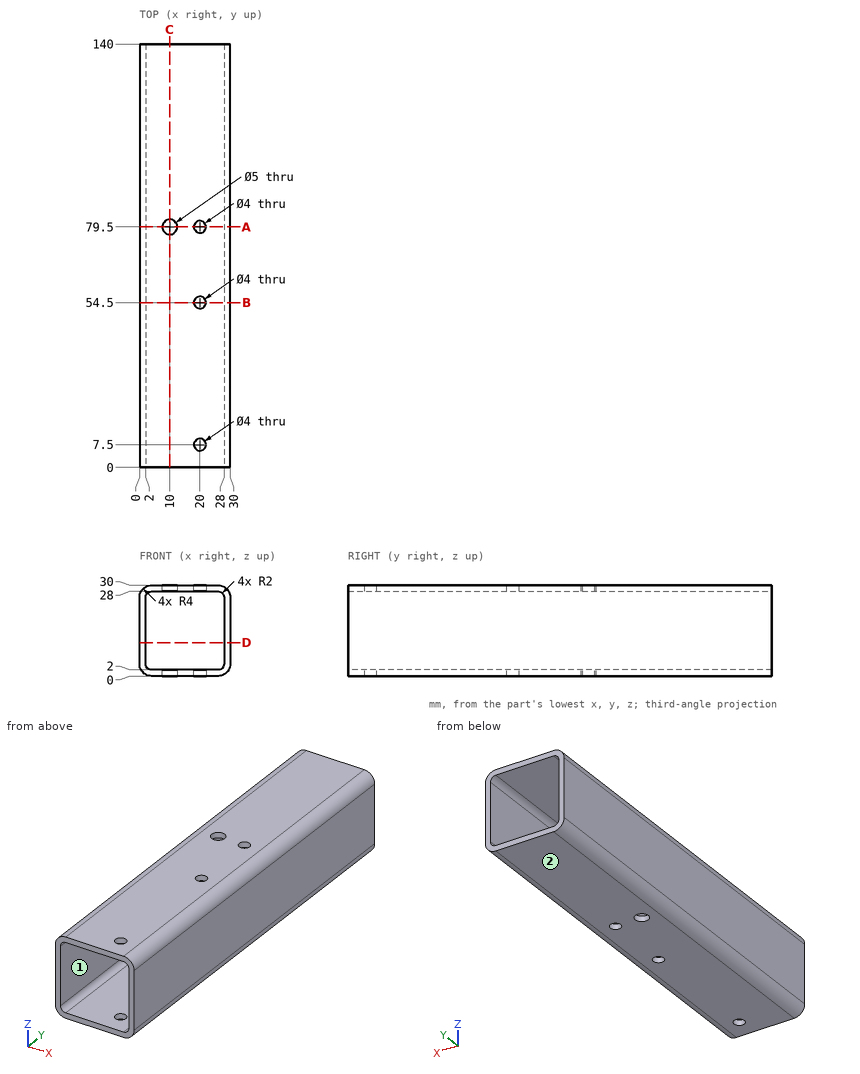
Job drawing, mm, ordinate dimensions from the low corner. One solid piece. A direction names the side the tool comes from. Give positions to 0.01 mm unless a question says otherwise; leave off trailing zeros. Write each loop counter-clockwise with the first axis right and the second up, starting at its lowest first coordinate (ties: lowest second). Pieces come first, ordered by that corner, then holes. Notation, with made-up numbers: (33, 3.25) -> (43, 3.25) arc R9 ccw to (43, 10.25) -> close; hole circle Ø1 at (9.25, -5). An arc over 180 degrees is marked (long way). Return JSON: item names as keys, results as strings.
Item 1: Band-saw the part on D-D (z = 11). List the corners of the cut face in (x, y).
Answer below:
{"outline": "(0, 0) -> (2, 0) -> (2, 140) -> (0, 140) -> close; (28, 0) -> (30, 0) -> (30, 140) -> (28, 140) -> close"}
Item 2: Drill centre lines: probe 1 along Y at (x, z) = (20, 29.25); probe 2 along Y at (x, z) = (10, 29.1); probe 3 along Z at (x, y) = (10.5, 38). Where is each one in solid material? Low to high.
Answer below:
{"probe 1": "y = 0 to 5.5, 9.5 to 52.5, 56.5 to 77.5, 81.5 to 140", "probe 2": "y = 0 to 77, 82 to 140", "probe 3": "z = 0 to 2, 28 to 30"}
Item 3: Band-saw the part on B-B (y = 54.5). List the corners of the cut face in (x, z), then the cut area to 3 significant figures.
Answer below:
{"outline": "(0, 4) arc R4 ccw to (4, 0) -> (18, 0) -> (18, 2) -> (4, 2) arc R2 cw to (2, 4) -> (2, 26) arc R2 cw to (4, 28) -> (18, 28) -> (18, 30) -> (4, 30) arc R4 ccw to (0, 26) -> close; (22, 0) -> (26, 0) arc R4 ccw to (30, 4) -> (30, 26) arc R4 ccw to (26, 30) -> (22, 30) -> (22, 28) -> (26, 28) arc R2 cw to (28, 26) -> (28, 4) arc R2 cw to (26, 2) -> (22, 2) -> close", "area": "198 mm2"}
Item 4: Band-saw the part on A-A (y = 79.5). Give the number of separate pieces and of enclosed holes in the cut face, then the cut area to 3 significant figures.
Answer below:
{"separate pieces": "4", "enclosed holes": "0", "area": "178 mm2"}
Item 5: Band-saw the part on C-C (x = 10). List the corners of the cut face in (y, z), then the cut area to 3 significant figures.
Answer below:
{"outline": "(0, 0) -> (77, 0) -> (77, 2) -> (0, 2) -> close; (0, 28) -> (77, 28) -> (77, 30) -> (0, 30) -> close; (82, 0) -> (140, 0) -> (140, 2) -> (82, 2) -> close; (82, 28) -> (140, 28) -> (140, 30) -> (82, 30) -> close", "area": "540 mm2"}
Item 6: Tool access for the marked faces 1 and 2: list every direction of +Z, -Z, +X, -X, +Y, -Y with a clear straight run to the whole face (end or side of a thin tool).
Answer below:
{"face 1": "+Y, -Y", "face 2": "-Z, +X, -X, +Y, -Y"}
